CAD build for the part. Positions are in the model's coordinates, mm. A direction names the side the tool comes from. Give positions to 0.01 mm unless a question says otherwise; leave off trailing zeros. Order: outer loops, then holes, each group sorted by start corner. A loop starts at its lowest first (then second) coordinate and runs counter-clockwise, first axis right, second up. Notation, with made-up numbers: (52, 88) -> (84, 88) arc R21 ccw to (84, 97) -> close; hole circle Ø3 at (-3.75, 13.5). An arc over 180 degrees is marked (long way). Answer as CSV lines item,"result".
```python
from build123d import *

# Parameters (mm, degrees)
SM_BASE_FLANGE_1_DEPTH = 50
SKETCH_3_R             = 6.5
CUT_EXTRUDE_2_DEPTH    = 74.464277033
CHAMFER_1_SIZE         = 3
CUT_EXTRUDE_3_DEPTH    = 74.464277033
PATTERN_LINEAR_1_COUNT = 2
PATTERN_LINEAR_1_PITCH = 30


# Sheet-metal steps are written as plain solids
with BuildPart() as part:
    # Sketch 1 → 基材-凸緣1 (new body)
    with BuildSketch(Plane(origin=(0, 0, 0), x_dir=(1, 0, 0), z_dir=(0, 1, 0))):
        with BuildLine():
            Line((31, 0), (4.7366, 0))
            ThreePointArc((4.7366, 0), (1.38731802, 1.38731802), (0, 4.7366))
            Line((0, 4.7366), (0, 44))
            Line((0, 44), (4, 44))
            Line((4, 44), (4, 4.7366))
            ThreePointArc((4, 4.7366), (4.215745145, 4.215745145), (4.7366, 4))
            Line((4.7366, 4), (31, 4))
            Line((31, 4), (31, 0))
        make_face()
    extrude(amount=SM_BASE_FLANGE_1_DEPTH)

    # Sketch 3 → 除料-伸長2 (cut, through all)
    with BuildSketch(Plane.ZY):
        with Locations((-22.7366, 25)):
            Circle(SKETCH_3_R)
    extrude(amount=-CUT_EXTRUDE_2_DEPTH, mode=Mode.SUBTRACT)

    # 導角1
    chamfer_1_edges = [part.edges().sort_by_distance(p)[0] for p in [
        (31, 50, -2),
        (31, 0, -2),
        (2, 50, -44),
        (2, 0, -44),
    ]]
    chamfer(chamfer_1_edges, length=CHAMFER_1_SIZE)

    # 草圖4 → 除料-伸長3 (cut, through all)
    with BuildSketch(Plane.XY):
        with BuildLine():
            Line((24.6, 7.4), (19.6, 7.4))
            ThreePointArc((19.6, 7.4), (17, 10), (19.6, 12.6))
            Line((19.6, 12.6), (24.6, 12.6))
            ThreePointArc((24.6, 12.6), (27.2, 10), (24.6, 7.4))
        make_face()
    cut_extrude_3 = extrude(amount=-CUT_EXTRUDE_3_DEPTH, mode=Mode.SUBTRACT)

    # 直線複製排列1: 除料-伸長3 ×2
    with Locations(*[(0, i * PATTERN_LINEAR_1_PITCH, 0) for i in range(1, PATTERN_LINEAR_1_COUNT)]):
        add(cut_extrude_3, mode=Mode.SUBTRACT)


solid = part.part
```
1) Band-saw the part on C-C, the plane x = 3. Write the cut outline in (y, z).
Data:
outline,"(0, -41) -> (3, -44) -> (47, -44) -> (50, -41) -> (50, -0.33) -> (0, -0.33) -> close; hole circle Ø13 at (25, -22.74)"
2) Band-saw the part on B-B, the plane y = 45.5. Write the cut outline in (x, z).
Data:
outline,"(0, -44) -> (4, -44) -> (4, -4.74) arc R0.74 cw to (4.74, -4) -> (31, -4) -> (31, 0) -> (4.74, 0) arc R4.74 ccw to (0, -4.74) -> close"
3) Band-saw the part on A-A, the plane y = 25. Write the cut outline in (x, z), then the cut area to 3 significant figures.
Data:
outline,"(0, -44) -> (4, -44) -> (4, -29.24) -> (0, -29.24) -> close; (0, -16.24) -> (4, -16.24) -> (4, -4.74) arc R0.74 cw to (4.74, -4) -> (31, -4) -> (31, 0) -> (4.74, 0) arc R4.74 ccw to (0, -4.74) -> close"
area,"227 mm2"
4) Pull direction X, two halves, no side cores. Call faces 1 (the flat face through (18, 25, -4)), 2 (the flat face through (22, 42.6, -2)), 3 (the flat face through (29, 1, -2)): pulls with the +X half, pulls with the -X half, needs draft (parallel to the pull), parting line crosses it, or undercut.
Data:
face 1,"needs draft"
face 2,"undercut"
face 3,"pulls with the +X half"
5) Wall check: line 1 along X through (y, z) = (28, -33); line 2 along Y through (x, z) = (2.5, -27); line 3 along Z through (x, y) = (5, 37). Give the ranges that are in metal, low to high. Write a range as [from, to].
Data:
line 1,"x = [0, 4]"
line 2,"y = [0, 20.09], [29.91, 50]"
line 3,"z = [-4, 0]"
6) Pin check, flat tips, straight feed: P1, Ø5, axis at y = 11, z = -9.5, coming from the +X side; P2, Ø4, axis at x = 10, y = 16, coming from the -Z side. Stop position of each tip, or through.
Data:
P1,"stops at x = 4"
P2,"stops at z = -4"
7) Band-saw the part on D-D, the plane y = 40. Write the cut outline in (x, z).
Data:
outline,"(0, -44) -> (4, -44) -> (4, -4.74) arc R0.74 cw to (4.74, -4) -> (17, -4) -> (17, 0) -> (4.74, 0) arc R4.74 ccw to (0, -4.74) -> close; (27.2, -4) -> (31, -4) -> (31, 0) -> (27.2, 0) -> close"
8) Which spindle directions (+Z, -Z, +X, -X, +Y, -Y) get a long thin tool onto all of the face, cutting with end or side? Do faces 4 (the flat face through (2, 2, -43)), 5 (the cylindrical face through (27.2, 10.1, -2)), 6 (the flat face through (4, 19, -29)). Say none if no direction does.
Data:
face 4,"-Z, +X, -X, -Y"
face 5,"+Z, -Z"
face 6,"-Z, +X, +Y, -Y"
